Can you work these out from the model? Positions are in its coordinate system, mm. A direction names the side the tool comes from. Give positions to 0.01 mm unless a question says otherwise; leave off trailing zeros. Order: outer loops, then holes, each group sorted by start corner. A loop starts at its lowest first (then second) coordinate and runs counter-clockwise, first axis right, second up. Notation, with made-up numbers: M 81,-1 L 132,-1 A26 cw 132,25 Z; hole C -15,15 d9. An arc over 180 degrees is marked long. Write each question's results on one line, items separated by ' | '.
Autodesk Inventor part; units mm, degrees
ref_plane "YZ Plane" through (0, 0, 0) normal (1, 0, 0) x (0, 1, 0)
ref_plane "XZ Plane" through (0, 0, 0) normal (0, 1, 0) x (-1, 0, 0)
ref_plane "XY Plane" through (0, 0, 0) normal (0, 0, 1) x (1, 0, 0)
sketch "Sketch2" plane through (0, 0, 0) normal (0, 0, 1) x (1, 0, 0)
  line L0 (-18, 5) -> (18, 5)
  line L1 (18, 5) -> (18, -5)
  line L2 (18, -5) -> (-18, -5)
  line L3 (-18, -5) -> (-18, 5)
  line L4 (-18, 5) -> (18, -5) construction
  line L5 (18, 5) -> (-18, -5) construction
  point P0 (0, 0)
  dimension "d0" = 10
  dimension "d1" = 36
extrude "Extrusion1" add sketch "Sketch2" along normal blind 11
sketch "Sketch3" plane through (0, 0, 11) normal (0, 0, 1) x (1, 0, 0)
  line L0 (-15.6, 12.15) -> (15.6, 12.15)
  line L1 (15.6, 12.15) -> (15.6, -12.15)
  line L2 (15.6, -12.15) -> (-15.6, -12.15)
  line L3 (-15.6, -12.15) -> (-15.6, 12.15)
  line L4 (-15.6, 12.15) -> (15.6, -12.15) construction
  line L5 (15.6, 12.15) -> (-15.6, -12.15) construction
  point P0 (0, 0)
  dimension "d4" = 31.2
  dimension "d5" = 24.3
extrude "Extrusion2" cut sketch "Sketch3" against normal blind 1
sketch "Sketch4" plane through (0, 0, 10) normal (0, 0, 1) x (1, 0, 0)
  circle A0 centre (12.5, 0) radius 1.65
  line L0 (0, 0) -> (0, 4.6535) construction
  circle A1 centre (-12.5, 0) radius 1.65
  point P0 (-61.5247, -30.2854)
  point P1 (15.4586, -30.2854)
  dimension "d39" = 3.3
  dimension "d40" = 25
extrude "Extrusion3" cut sketch "Sketch4" against normal through all
sketch "Sketch7" plane through (0, 0, 11) normal (0, 0, 1) x (1, 0, 0)
  arc A0 (21.3831, -3.7533) -> (21.3831, 3.7533) centre (20, 0) ccw
  line L0 (21.3831, 3.7533) -> (18, 5)
  line L1 (18, 5) -> (18, -5)
  line L2 (18, -5) -> (21.3831, -3.7533)
  line L3 (0, 20.7674) -> (0, -20.7674) construction
  arc A1 (-21.3831, 3.7533) -> (-21.3831, -3.7533) centre (-20, 0) ccw
  line L4 (-21.3831, 3.7533) -> (-18, 5)
  line L5 (-18, 5) -> (-18, -5)
  line L6 (-18, -5) -> (-21.3831, -3.7533)
  line L7 (18, -5) -> (18, 5) construction
  circle A2 centre (20, 0) radius 1.65
  circle A3 centre (-20, 0) radius 1.65
  line L8 (0, 0) -> (1.9739, 0) construction
  dimension "d28" = 3.3
  dimension "d29" = 4
  dimension "d30" = 40
  dimension "d31" = 10
extrude "Extrusion6" add sketch "Sketch7" against normal up to surface (11 mm away)
sketch "Sketch9" plane through (0, 0, 10) normal (0, 0, 1) x (1, 0, 0)
  circle A0 centre (-12.5, 0) radius 1.65
  line L0 (-9.3246, 0) -> (-10.9123, -2.75)
  line L1 (-10.9123, -2.75) -> (-14.0877, -2.75)
  line L2 (-14.0877, -2.75) -> (-15.6754, 0)
  line L3 (-15.6754, 0) -> (-14.0877, 2.75)
  line L4 (-14.0877, 2.75) -> (-10.9123, 2.75)
  line L5 (-10.9123, 2.75) -> (-9.3246, 0)
  line L6 (0, 0) -> (0, 3.6506) construction
  circle A1 centre (12.5, 0) radius 1.65
  line L7 (9.3246, 0) -> (10.9123, -2.75)
  line L8 (10.9123, -2.75) -> (14.0877, -2.75)
  line L9 (14.0877, -2.75) -> (15.6754, 0)
  line L10 (15.6754, 0) -> (14.0877, 2.75)
  line L11 (14.0877, 2.75) -> (10.9123, 2.75)
  line L12 (10.9123, 2.75) -> (9.3246, 0)
  dimension "d41" = 5.5
extrude "Extrusion8" cut sketch "Sketch9" against normal blind 2.5
sketch "Sketch8" plane through (0, 0, 0) normal (1, 0, 0) x (0, 1, 0)
  line L0 (45.1511, -28.2394) -> (-45.1511, -28.2394)
  line L1 (-45.1511, -28.2394) -> (-45.1511, 28.2394)
  line L2 (-45.1511, 28.2394) -> (45.1511, 28.2394)
  line L3 (45.1511, 28.2394) -> (45.1511, -28.2394)
  line L4 (45.1511, -28.2394) -> (-45.1511, 28.2394) construction
  line L5 (-45.1511, -28.2394) -> (45.1511, 28.2394) construction
  point P0 (0, 0)
extrude "Extrusion7" cut sketch "Sketch8" along normal blind 24 and the other way blind 9
properties part number "power_signal_socket_fixed3" material "Acetal Resin, Black"
(1) Will this pin go through, and if not, where does the flat tip stop? P1, Ø1.5, axis at y = 1, z = 4, coming from the -X side.
Data:
P1: stops at x = -23.99
(2) Imagine slicing it at B-B, the plane z = 4.5. Write out the boundary of the cut face in (x, y), plus the area to 3 significant figures.
Data:
outline: M -21.38,-3.75 L -18,-5 L -9,-5 L -9,5 L -18,5 L -21.38,3.75 A4 ccw Z; hole C -20,0 d3.3; hole C -12.5,0 d3.3 | area: 117 mm2
(3) For faces 4 (the face through (-13, 2.75, 9)), 5 (the face through (-15.6, -0.1, 10.5)), 6 (the face through (-19.668, -4.385, 5.577)), which set-ups out of +Z, -Z, +X, -X, +Y, -Y let a thin tool reach every point of the face, with its end or its side?
Data:
face 4: +Z | face 5: +Z, +X, +Y, -Y | face 6: +Z, -Z, -X, -Y
(4) I need wall thicknesses on L1, parallel to Y at x = -12, z = 9.25; L2, parallel to Y at x = -12.5, z = 4.75; L3, parallel to Z at x = -14.5, y = -3.75. Which ranges of each line are inside material? Lowest first, please. Write a range as from..to.
Data:
L1: y = -5..-2.75, 2.75..5 | L2: y = -5..-1.65, 1.65..5 | L3: z = 0..10
(5) Imagine slicing it at D-D, the plane z = 8. Write out the boundary of the cut face in (x, y), plus the area to 3 significant figures.
Data:
outline: M -21.38,-3.75 L -18,-5 L -9,-5 L -9,5 L -18,5 L -21.38,3.75 A4 ccw Z; hole C -20,0 d3.3; hole M -15.68,0 L -14.09,-2.75 L -10.91,-2.75 L -9.32,0 L -10.91,2.75 L -14.09,2.75 Z | area: 99.2 mm2
(6) Imagine slicing it at C-C, the plane y = 3.25. Write out the boundary of the cut face in (x, z), plus the area to 3 significant figures.
Data:
outline: M -22.33,0 L -9,0 L -9,10 L -15.6,10 L -15.6,11 L -22.33,11 Z | area: 140 mm2
(7) Imagine slicing it at A-A, the plane x = -12.5. Write out the boundary of the cut face in (y, z).
Data:
outline: M -5,0 L -1.65,0 L -1.65,7.5 L -2.75,7.5 L -2.75,10 L -5,10 Z; M 1.65,0 L 5,0 L 5,10 L 2.75,10 L 2.75,7.5 L 1.65,7.5 Z
(8) We'd pull the mould along X, two halves only. Please class faces 1 (the face through (-24, 0, 6)), 2 (the face through (-10.976, -0.632, 3.802)), 3 (the face through (-14, 5, 5)): +X half, -X half, draft (parallel to the pull), parting line (faces both ways), or undercut.
Data:
face 1: -X half | face 2: undercut | face 3: draft
